Answer from the drawing. Dimensions are ordinates in mm from the lowest x, y and z of the part. Give positions to 0.01 mm unless a question says otherwise; leave off trailing zeros. Loops run counter-clockwise (first coordinate to the right, second up) from the corner with the lowest first, then second, coordinate; pieces in that order, holes last.
Item 1: Section D-D, the plane x = 33.85 is taken. Give the vertices of the cut face in (y, z).
Item 2: Section A-A, the plane z = 49 is taken. Give the vertices of the cut face in (x, y), and give its area (3 significant figures).
Item 3: Section B-B, the plane y = 0.5 is taken. Give the number of separate pieces and of enclosed holes in the cut face, and give its area (3 significant figures).
Item 4: Consider line 1 along Z through (x, y) = (77, 1.5); line 2 along Z through (x, y) = (90.5, 0.4); line 3 along Z through (x, y) = (5.25, 0.5). Determine where each line is inside the solid, lowest interval first.
Item 5: Each of these flat-tipped pins is pushed along its axis until it touches: pin 1 Ø1.5 at (x, z) = (76.9, 94.75) entering from +Y; pin 2 Ø0.6 at (x, y) = (20, 1) entering from +Z. Where does it stop, or does it pass through?
Item 6: Section C-C, the plane z = 23.4 is taken. Give the vertices of the cut face in (x, y), and give its area (3 significant figures).
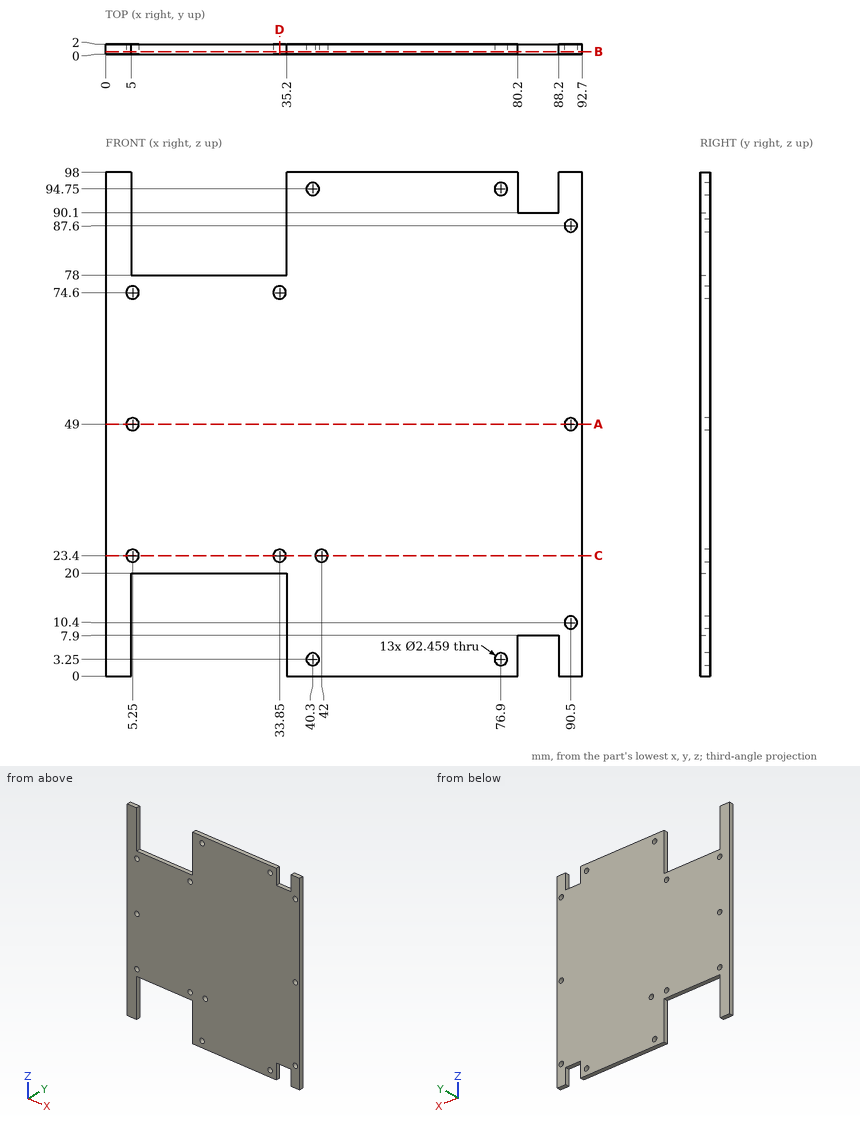
Worked answers:
1. outline: (0, 20) - (2, 20) - (2, 22.17) - (0, 22.17) - close; (0, 24.63) - (2, 24.63) - (2, 73.37) - (0, 73.37) - close; (0, 75.83) - (2, 75.83) - (2, 78) - (0, 78) - close
2. outline: (0, 0) - (4.02, 0) - (4.02, 2) - (0, 2) - close; (6.48, 0) - (89.27, 0) - (89.27, 2) - (6.48, 2) - close; (91.73, 0) - (92.7, 0) - (92.7, 2) - (91.73, 2) - close
2. area: 176 mm2
3. separate pieces: 1
3. enclosed holes: 13
3. area: 7,690 mm2
4. line 1: z = 0 to 2.02, 4.48 to 93.52, 95.98 to 98
4. line 2: z = 0 to 9.17, 11.63 to 47.77, 50.23 to 86.37, 88.83 to 98
4. line 3: z = 20 to 22.17, 24.63 to 47.77, 50.23 to 73.37, 75.83 to 78
5. pin 1: passes through
5. pin 2: stops at z = 78
6. outline: (0, 0) - (4.02, 0) - (4.02, 2) - (0, 2) - close; (6.48, 0) - (32.62, 0) - (32.62, 2) - (6.48, 2) - close; (35.08, 0) - (40.77, 0) - (40.77, 2) - (35.08, 2) - close; (43.23, 0) - (92.7, 0) - (92.7, 2) - (43.23, 2) - close
6. area: 171 mm2
